Part model, mm, in its own coordinate system. Face numbers are marked on the shaded views. A direction names the side the tool comes from. Round coordinates to 2 decimals unless told otherwise and drop trailing zeros. Order: outer loops, then holes, each group sorted by start corner. A loop starts at its lowest first (then second) coordinate and runs counter-clockwise, first axis right, second up. Notation, with made-up numbers: (10.25, 34) - (23.25, 34) arc R17 ccw to (23.25, 57) - close; hole circle Ø8 at (-24.5, 33). An arc over 180 degrees is marked (long way). Return JSON: item names as keys, results as strings. Group by question number.
Item 1: Saw through at B-B on z = 38. List the corners of the cut face in (x, y).
Item 2: Saw through at A-A on y = 30. State how many separate pieces and enclosed holes the cut face has, and give its area (3 significant figures).
Item 3: Probe probe 1 along X at (y, z) = (32, 15); probe 2 along X at (y, z) = (-31.5, 7.5); probe 3 along Z at (x, y) = (-33.6, 30). List the from-to ranges inside material, lowest first.
Item 4: Drop flat-ended pins along their axis: pin 1 (1.6 mm diameter, centred on x = -26, y = 38.5, fed in from +Z); pin 2 (5 mm diameter, centred on x = -15.5, z = 60, fed in from -Y); pin 3 (5 mm diameter, centred on y = 2, z = 16, fed in from +X); pin 4 (8.5 mm diameter, centred on x = -27, y = -6.5, fed in from +Z). Give the stop position or say it passes through.
Item 5: Two-plate mould, pull along Z, no slides. Class the marked faces 5, 6 and 7: released by +Z, released by -Z, zero draft, split by the parting line, or undercut.
Item 6: Tool access for the marked faces 1, 2, 3 and 4: list every direction of +Z, -Z, +X, -X, +Y, -Y with a clear straight run to the whole face (end or side of a thin tool).
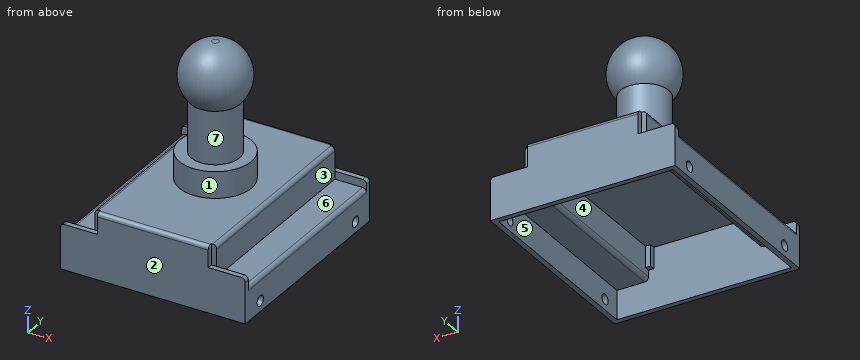
```python
from build123d import *

# Parameters (mm, degrees)
F1_W      = 70
F1_H      = 25
F2_DEPTH  = 78.5
F3_W      = 15
F3_H      = 10
F4_DEPTH  = 2
F5_W      = 15
F5_H      = 10
F6_DEPTH  = 2
F7_W      = 17.4621326589
F7_H      = 19.2356310288
F8_DEPTH  = 74.5
F10_T     = -2
F11_R     = 1.5
F12_R     = 1.95
F13_DEPTH = 70.001
F14_R     = 13.6
F15_DEPTH = 10
F16_R     = 9.1
F17_DEPTH = 20
F18_R     = 12.5
F19_DEPTH = 21


# Not quite as in the source:
# - a feature of the source that left no trace in its solid (it failed there, or was rolled back) is left out


with BuildPart() as f2:
    # F1 (on offset) → F2 (new body)
    with BuildSketch(Plane.XZ.offset(39.5)):
        with Locations((0, 12.5)):
            Rectangle(F1_W, F1_H)
    extrude(amount=-F2_DEPTH)

    # F3 (on face) → F4 (cut)
    with BuildSketch(Plane.XZ.offset(39.5)):
        with Locations((-28.5, 22)):
            Rectangle(F3_W, F3_H)
        with Locations((28.5, 22)):
            Rectangle(F3_W, F3_H)
    extrude(amount=-F4_DEPTH, mode=Mode.SUBTRACT)

    # F5 (on face) → F6 (cut)
    with BuildSketch(Plane(origin=(0, 39, 0), x_dir=(-1, 0, 0), z_dir=(0, 1, 0))):
        with Locations((-28.5, 21)):
            Rectangle(F5_W, F5_H)
        with Locations((28.5, 21)):
            Rectangle(F5_W, F5_H)
    extrude(amount=-F6_DEPTH, mode=Mode.SUBTRACT)

    # F7 (on face) → F8 (cut)
    with BuildSketch(Plane.XZ.offset(37.5)):
        with Locations((-31.7310663294, 22.6178155144)):
            Rectangle(F7_W, F7_H)
        with Locations((31.7310663294, 22.6178155144)):
            Rectangle(F7_W, F7_H)
    extrude(amount=-F8_DEPTH, mode=Mode.SUBTRACT)

    # F10: a shell. OpenCascade refuses it in one call, so the cavity is built on its own and cut out:
    # the body offset inwards by the wall thickness, plus a prism from it out through each open face.
    f10_core = offset(f2.part, amount=F10_T, kind=Kind.INTERSECTION, mode=Mode.PRIVATE)
    f10_exits = [f10_core.faces().sort_by_distance(p)[0] for p in [
        (0, -0.25, 2),
    ]]
    add(f10_core, mode=Mode.SUBTRACT)
    extrude(f10_exits, amount=-F10_T, mode=Mode.SUBTRACT)

    # F11
    f11_edges = [f2.edges().sort_by_distance(p)[0] for p in [
        (21, -0.25, 11),
        (-21, -0.25, 11),
        (-35, -38.5, 17),
        (-35, 38, 16),
        (-35, -0.25, 13),
        (-23, -0.25, 25),
        (0, -39.5, 25),
        (0, 39, 25),
        (23, -0.25, 25),
        (35, -38.5, 17),
        (35, -0.25, 13),
        (35, 38, 16),
    ]]
    fillet(f11_edges, radius=F11_R)

    # F12 (on face) → F13 (cut, through all)
    with BuildSketch(Plane.YZ.offset(35)):
        with Locations((-30, 4)):
            Circle(F12_R)
        with Locations((30, 4)):
            Circle(F12_R)
    extrude(amount=-F13_DEPTH, mode=Mode.SUBTRACT)

    # F14 (on face) → F15 (join)
    with BuildSketch(Plane.XY.offset(25)):
        Circle(F14_R)
    extrude(amount=F15_DEPTH)

    # F16 (on face) → F17 (join)
    with BuildSketch(Plane.XY.offset(35)):
        Circle(F16_R)
    extrude(amount=F17_DEPTH)

    # F18 (on face) → F19 (join)
    with BuildSketch(Plane.XY.offset(55)):
        Circle(F18_R)
    extrude(amount=F19_DEPTH)

    # F20 (on Front) → F21 (revolve, cut)
    with BuildSketch(Plane.XZ):
        with BuildLine():
            ThreePointArc((0, 76.0678347956), (11.4737550942, 68.5243920963), (9.100375697, 54.9996867776))
            Line((9.100375697, 54.9996867776), (14.105156064, 54.9996867776))
            Line((14.105156064, 54.9996867776), (14.105156064, 76.9773796201))
            Line((14.105156064, 76.9773796201), (0, 76.9773796201))
            Line((0, 76.9773796201), (0, 76.0678347956))
        make_face()
    revolve(axis=Axis((0, 0, 76.5226072078), (0, 0, -1)), mode=Mode.SUBTRACT)


solid = f2.part
```
Filled in:
{
 "1": {"outline": "circle Ø18.2 at (0, 0)"},
 "2": {"separate pieces": "3", "enclosed holes": "0", "area": "214 mm^2"},
 "3": {"probe 1": "x = -23 to -21, 21 to 23", "probe 2": "x = -35 to -33, 33 to 35", "probe 3": "z = 0 to 2.05, 5.95 to 13"},
 "4": {"pin 1": "stops at z = 16", "pin 2": "passes through", "pin 3": "stops at x = 23", "pin 4": "stops at z = 24.33"},
 "5": {"face 5": "zero draft", "face 6": "released by +Z", "face 7": "undercut"},
 "6": {"face 1": "+Z", "face 2": "+Z, -Z, +X, -X, -Y", "face 3": "+Z, +X", "face 4": "-Z"}
}
